The figure shows three views and two pictorial views of one solid part (mm, origin at its lowest corner). Answer the questions. A direction names the side the tool comes from. Coordinates: 2 decimals unless noted, no trailing zeros. Write each loop counter-clockwise with the first axis right and the second up, starting at its lowest first coordinate (ties: lowest second). Pieces come first, ordered by that corner, then holes. Notation, with made-up numbers: M 88,42 L 100,42 A22 ccw 100,60 Z; hole C 8.25,49 d7. An arc over 180 degrees is marked long. Write item = value, one per line. Start each with the question number.
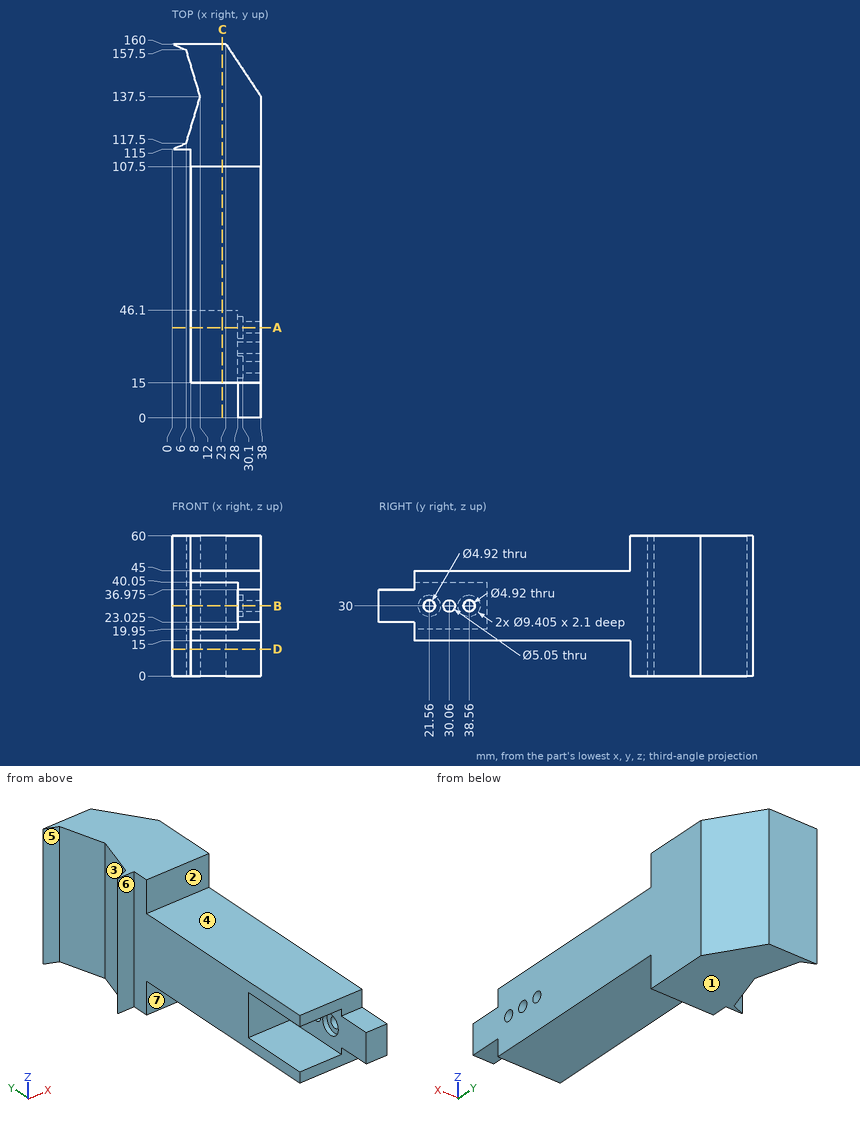
1. The part is cut by section D-D, the plane z = 11.5. Write down the section's boundary in (x, y).
2. The part is cut by section B-B, the plane z = 30. Count the separate pieces of the cut face and the enclosed holes in it, and give its area (3 significant figures).
3. The part is cut by section C-C, the plane x = 21.5. Write down the section's boundary in (y, z).
4. Each of these flat-tipped pins is pushed along its axis until it touches: pin 1 (6 mm diameter, centred on x = 16, z = 33, fed in from -Y); pin 2 (3 mm diameter, centred on x = 26, z = 30.5, fed in from +Y); pin 3 (1 mm diameter, centred on x = 23, y = 19, fed in from -Z). Where does it stop, or does it pass through?
5. For the marked faces 4, 5, 6 and 7, determine the directions among +Z, -Z, +X, -X, +Y, -Y from which every point of the face is accessible in a straight line to the end or side of a thin tool.
6. Straight lines are drawn through the part: L1, parallel to Z at x = 34.5, y = 21.56; L2, parallel to Y at x = 29.6, z = 30 (1 decimal); L3, parallel to Y at x = 35.25, z = 30 (3 decimals). For each, find the intervals that lie inside material, in ascending order. Write a range as [from, to].
7. The part is cut by section A-A, the plane y = 38.56. Write down the section's boundary in (x, z), and give its area (3 significant figures).
8. For a pull along Y with two mould halves and no side action, classify the marked faces 1, 2 and 3 as pulls with the +Y half, pulls with the -Y half, needs draft (parallel to the pull), parting line crosses it, or undercut.
Solution:
q1.outline = M 0,115 L 8,115 L 8,107.5 L 38,107.5 L 38,137.5 L 23,160 L 0,160 L 6,157.5 L 12,137.5 L 6,117.5 Z
q2.separate_pieces = 4
q2.enclosed_holes = 0
q2.area = 3,530 mm^2
q3.outline = M 15,15 L 107.5,15 L 107.5,0 L 160,0 L 160,60 L 107.5,60 L 107.5,45 L 15,45 L 15,40.05 L 46.1,40.05 L 46.1,19.95 L 15,19.95 Z
q4.pin_1 = 46.1
q4.pin_2 = 157.75
q4.pin_3 = 15
q5.face_4 = +Z, +X, -X, -Y
q5.face_5 = +Z, -Z, -X
q5.face_6 = +Z, -Z, -X, -Y
q5.face_7 = -Z, +X, -X, -Y
q6.L1 = [15, 27.54], [32.46, 45]
q6.L2 = [0, 16.9], [26.3, 27.5], [32.6, 33.9], [43.3, 150.1]
q6.L3 = [0, 19.1], [24.02, 27.535], [32.585, 36.1], [41.02, 141.625]
q7.outline = M 8,15 L 38,15 L 38,27.54 L 30.1,27.54 L 30.1,25.3 L 28,25.3 L 28,19.95 L 8,19.95 Z; M 8,40.05 L 28,40.05 L 28,34.7 L 30.1,34.7 L 30.1,32.46 L 38,32.46 L 38,45 L 8,45 Z
q7.area = 439 mm^2
q8.face_1 = needs draft
q8.face_2 = pulls with the -Y half
q8.face_3 = undercut
